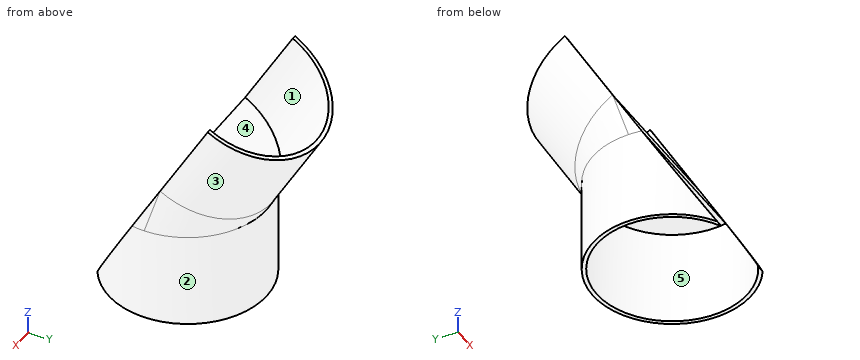
Autodesk Inventor part; units mm, degrees
ref_plane "Work Plane3" through (11.7088, 33.02, 42.8397) normal (0, 0.5, 0.8660254) x (-1, 0, 0)
ref_plane "Work Plane4" through (0.2515, -1.9323, 107.0135) normal (0, -0.8660254, 0.5) x (1, 0, 0)
ref_plane "YZ Plane" through (0, 0, 0) normal (1, 0, 0) x (0, 1, 0)
sketch "Sketch1" plane through (0, 0, 0) normal (0, 0, 1) x (1, 0, 0)
  circle A0 centre (0, 0) radius 31.75
  dimension "d0" = 63.5
extrude "Extrusion1" add sketch "Sketch1" along normal blind 38.1
sketch "Sketch2" plane through (0, 0, 38.1) normal (0, 0, 1) x (1, 0, 0)
  circle A0 centre (0, 0) radius 31.75
  point P0 (0, 31.75)
ref_plane "Work Plane1" through (0, 31.75, 38.1) normal (0, 1, 0) x (-1, 0, 0)
sketch "Sketch3" plane through (0, 31.75, 38.1) normal (0, 1, 0) x (-1, 0, 0)
  line L0 (-11.7088, 2.54) -> (14.1872, 2.54) construction
  line L1 (31.75, 0) -> (-31.75, 0)
  point P0 (0, -38.1)
  dimension "d3" = 2.54
ref_plane "Work Plane3" through (11.7088, 33.02, 42.8397) normal (0, 0.5, 0.8660254) x (-1, 0, 0)
ref_plane "Work Plane2" through (11.7088, 31.75, 40.64) normal (0, 0.5, 0.8660254) x (-1, 0, 0)
sketch "Sketch5" plane through (11.7088, 33.02, 42.8397) normal (0, 0.5, 0.8660254) x (-1, 0, 0)
  circle A0 centre (11.4573, 30.6064) radius 31.75
  line L0 (0.2164, -1.1436) -> (24.8554, -1.1436) construction
  point P0 (11.7088, 7.1763)
  dimension "d15" = 63.5
  dimension "d16" = 31.75
extrude "Extrusion3" add sketch "Sketch5" along normal blind 38.1
loft "Loft1" add section 1 edges at (-31.75, 0, 38.1) section 2 edges at (32.0015, 6.5141, 58.1429)
sketch "Sketch6" plane through (0, 0, 0) normal (0, 0, -1) x (-1, 0, 0)
  circle A0 centre (0, 0) radius 31.75
  circle A1 centre (0, 0) radius 30.1625
  dimension "d23" = 60.325
extrude "Extrusion4" cut sketch "Sketch6" against normal blind 38.1 contours A1
sketch "Sketch7" plane through (0.2515, 25.5641, 91.1385) normal (0, 0.5, 0.8660254) x (1, 0, 0)
  circle A0 centre (0, 0) radius 31.75
  circle A1 centre (0, 0) radius 30.1625
  point P0 (-0.2515, 23.4301)
  dimension "d26" = 60.325
extrude "Extrusion5" cut sketch "Sketch7" against normal blind 38.1 contours A1
sketch "Sketch8" plane through (0.2515, 25.5641, 91.1385) normal (0, 0.5, 0.8660254) x (1, 0, 0)
  circle A0 centre (0, 0) radius 30.1625
  circle A1 centre (0, 0) radius 31.75
  point P0 (-0.2515, 23.4301)
  point P1 (0, -31.75)
ref_plane "Work Plane4" through (0.2515, -1.9323, 107.0135) normal (0, -0.8660254, 0.5) x (1, 0, 0)
sketch "Sketch9" plane through (0.2515, -1.9323, 107.0135) normal (0, -0.8660254, 0.5) x (1, 0, 0)
  line L0 (-48.3779, -109.4634) -> (50.7956, -109.4634)
  line L1 (50.7956, -109.4634) -> (50.7956, 8.7454)
  line L2 (50.7956, 8.7454) -> (-48.3779, 8.7454)
  line L3 (-48.3779, 8.7454) -> (-48.3779, -109.4634)
  point P0 (-0.2515, -91.7103)
extrude "cut" cut sketch "Sketch9" against normal blind 31.75
properties part number "sup-angled" material "PVC-Piping"
Here's how the part is built. I have some questions about the finished solid (model axes, mm). Face numbers are marked on the shaded views. A direction names the side the tool comes from. Coordinates: 2 decimals unless noted, no trailing zeros. Answer in a Markdown table with one row per item.
(1) On a 3-axis mill with a long thin cutter (end or side, diameter ignored), from which of +Z, -Z, +X, -X, +Y, -Y can I reach the whole of each face in a straight line? I mean the marked faces 4 and 5. Say none if no direction works.
Answer key:
| item | result |
|---|---|
| face 4 | +Z |
| face 5 | -Z |
(2) Will these pins go through, and if not, where does the flat tip stop? pin 1 Ø1 at (y, z) = (17, 37.5) entering from +X; pin 2 Ø5 at (x, z) = (23, 16) entering from -Y; pin 3 Ø10 at (x, z) = (-4, 45) entering from +Y.
Answer key:
| item | result |
|---|---|
| pin 1 | x = 27.13 |
| pin 2 | y = -19.25 |
| pin 3 | y = 38.22 |
(3) Thinking about a two-plate mould opening in Y: for the marked faces 1, 2 and 3, which applies, +Y half, -Y half, draft (parallel to the pull), parting line (faces both ways), or undercut?
Answer key:
| item | result |
|---|---|
| face 1 | undercut |
| face 2 | parting line |
| face 3 | +Y half |
(4) Please list where these lines run through material, in increasing order: probe 1 along X at (y, z) = (0, 11); probe 2 along Y at (x, z) = (0, 24); probe 3 along Y at (x, z) = (12.5, 49.5).
Answer key:
| item | result |
|---|---|
| probe 1 | -31.75 to -30.16, 30.16 to 31.75 |
| probe 2 | 30.16 to 31.75 |
| probe 3 | 1.53 to 21.48, 33.35 to 35.35 |
